Here's how the part is built. I have some questions about the finished solid (model axes, mm). Face numbers are marked on the shaded views. A direction names the side the tool comes from. Give positions to 0.01 mm unless a question says otherwise; leave off trailing zeros. Write each loop counter-clockwise with the first axis right and the second up, starting at its lowest first coordinate (ties: lowest second). Pieces come first, ordered by that corner, then holes. Notation, with made-up numbers: (-27.75, 65) - (13.25, 65) arc R5 cw to (13.25, 72) - close; hole circle Ø6 at (-27, -10). An arc over 180 degrees is marked (long way). Use one line per item in the form item = value. Start each with the question number.
from build123d import *

# Parameters (mm, degrees)
F0_W     = 38.0493849516
F0_H     = 19.1407520324
F1_DEPTH = 152.4


# Not quite as in the source:
# - ends of sketch curves that miss each other by under 0.0002 mm in the source are joined


with BuildPart() as f1:
    # F0 (on Front) → F1 (new body)
    with BuildSketch(Plane.XZ):
        with Locations((-9.5677897334, 9.5703760162)):
            Rectangle(F0_W, F0_H)
        with BuildLine():
            Line((9.4569027424, 19.1407520324), (9.4569027424, 0))
            Line((9.4569027424, 0), (9.4569027424, -19.074914977))
            Line((9.4569027424, -19.074914977), (15.8548746258, -19.074914977))
            ThreePointArc((15.8548746258, -19.074914977), (17.7121304526, -14.6721322023), (22.1616335674, -12.9297724811))
            Line((22.1616335674, -12.9297724811), (22.1616335674, -7.981513619))
            ThreePointArc((22.1616335674, -7.981513619), (26.6843883176, -6.1079115975), (28.5572540015, -1.5848518815))
            ThreePointArc((28.5572540015, -1.5848518815), (27.7056149725, 1.6028958779), (25.3783776729, 3.941914994))
            ThreePointArc((25.3783776729, 3.941914994), (24.8908493588, 8.4306069892), (28.559631396, 11.0623512867))
            Line((28.559631396, 11.0623512867), (28.695607532, 15.8877193117))
            ThreePointArc((28.695607532, 15.8877193117), (27.7740633897, 18.1849926711), (25.4908129573, 19.1407520324))
            Line((25.4908129573, 19.1407520324), (9.4569027424, 19.1407520324))
        make_face()
    extrude(amount=F1_DEPTH)


solid = f1.part
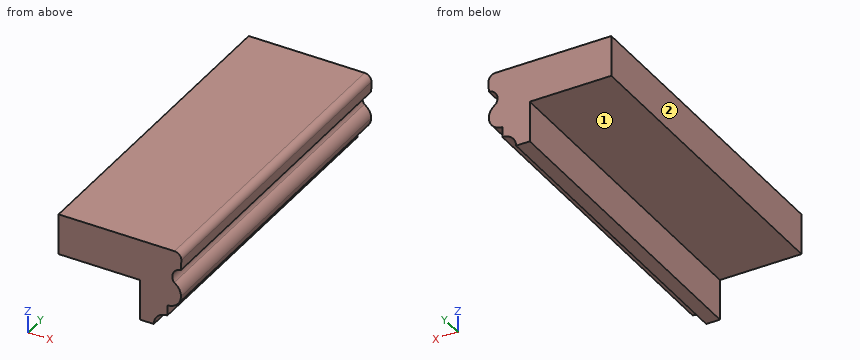
1. For P1, Ø6, axis at y = -81.5, z = -1, coming from the +X side; P2, Ø1.5, axis at y = -136, z = -13.5, coming from the -X side; P3, Ø2.5, axis at y = -56, z = -10, coming from the +X side, each with a flat end and sliding along its axis, tell me the tip position at first contact or that it passes through.
2. I want a section at C-C, the plane z = -6. List the corners of the cut face in (x, y) for me, then the cut area to 3 significant figures.
3. For the marked faces 1 and 2, which set-ups out of +Z, -Z, +X, -X, +Y, -Y let a thin tool reach every point of the face, with its end or its side?
4. I want a section at B-B, the plane x = -6. List the corners of the cut face in (y, z) for me, then the cut area to 3 significant figures.
5. Please list where these lines run through material, in increasing order: line 1 (Z direction, x = -8, y = -60); line 2 (X direction, y = -114, z = 7); line 3 (Z direction, x = 25.5, y = -141.5).
6. I want a section at A-A, the plane y = -131.5. List the corners of the cut face in (x, z) for me.
Result sheet:
q1.P1 = 28.56
q1.P2 = 9.46
q1.P3 = 22.16
q2.outline = (9.46, -152.4) - (26.79, -152.4) - (26.79, 0) - (9.46, 0) - close
q2.area = 2,640 mm2
q3.face_1 = -Z, -X, +Y, -Y
q3.face_2 = +Z, -Z, -X, +Y, -Y
q4.outline = (-152.4, 0) - (0, 0) - (0, 19.14) - (-152.4, 19.14) - close
q4.area = 2,920 mm2
q5.line_1 = 0 to 19.14
q5.line_2 = -28.59 to 24.52
q5.line_3 = -7.04 to 3.87, 9.42 to 19.14
q6.outline = (-28.59, 0) - (9.46, 0) - (9.46, -19.07) - (15.85, -19.07) arc R6.15 cw to (22.16, -12.93) - (22.16, -7.98) arc R6.4 ccw to (28.56, -1.58) arc R6.4 ccw to (25.38, 3.94) arc R4.48 cw to (28.56, 11.06) - (28.7, 15.89) arc R3.21 ccw to (25.49, 19.14) - (-28.59, 19.14) - close
